Source: CAD feature listing. Evaluate the final solid. Frame: model axes, mm. Coordinates: 2 decimals unless noted, no trailing zeros. Order: outer loops, then holes, each group sorted by start corner. A loop starts at its lowest first (then second) coordinate and runs counter-clockwise, first axis right, second up.
Item 1: Contact query for flat-ended pins moving along their axis: P1, Ø12, axis at x = 364, y = -477, coming from the +Z side; P2, Ø1, axis at x = 401.5, z = 6, coming from the -Y side; P3, Ø12, axis at x = 375.5, z = 83.5, coming from the +Y side. Output: stop coordinate, or through.
Item 2: Ray query, line 1 (Z direction, x = 364.5, y = 584); line 2 (Y direction, x = 385, z = 88); line 3 (Y direction, x = 375, z = 37). Return the intervals inside material, ascending.
Item 3: Mould query, pull axis Y, two halves, no side actions, for faces 1 (the flat face through (376, 816, 0)), 2 (the cylindrical face through (360.89, 829.51, 50.09)), 3 (the cylindrical face through (387.09, 794.28, 50.09)), 4 (the flat face through (356, 821, 101.6)). Classes: released by +Y, released by -Y, zero draft, split by the parting line, or undercut.
Item 4: Section A-A on x = 370. Return the cut outline in (y, z).
Item 5: Section B-B on y = 584.5. Return the cut outline in (x, z), then the cut area to 3 significant figures.
Item 6: Section C-C on z = 19. Return the cut outline in (x, y), then the cut area to 3 significant figures.
from build123d import *

# Parameters (mm, degrees)
F0_W     = 76.2
F0_H     = 2133.6
F1_DEPTH = 4.7625
F2_R     = 24.13
F2_R_2   = 20.447
F3_DEPTH = 101.6
F5_DEPTH = 35.814


with BuildPart() as f1:
    # F0 (on Top) → F1 (new body)
    with BuildSketch(Plane.XY):
        with Locations((375.958569, -213.009804)):
            Rectangle(F0_W, F0_H)
    extrude(amount=-F1_DEPTH)

    # F2 (on face) → F3 (join)
    with BuildSketch(Plane.XY):
        with Locations((375.958569, 815.690196)):
            Circle(F2_R)
        with Locations((375.958569, 815.690196)):
            Circle(F2_R_2, mode=Mode.SUBTRACT)
    extrude(amount=F3_DEPTH)

    # F4 (on face) → F5 (cut)
    with BuildSketch(Plane(origin=(0, 0, -4.7625), x_dir=(1, 0, 0), z_dir=(0, 0, -1))):
        Polygon((337.858569, 1107.854731), (414.058569, 1279.809804), (337.858569, 1279.809804), align=None)
    extrude(amount=-F5_DEPTH, mode=Mode.SUBTRACT)


solid = f1.part
Answer list:
1. P1: stops at z = 0
1. P2: passes through
1. P3: stops at y = 839.82
2. line 1: z = -4.76 to 0
2. line 2: y = 793.32 to 797.35, 834.03 to 838.06
2. line 3: y = 791.58 to 795.27, 836.11 to 839.8
3. face 1: undercut
3. face 2: undercut
3. face 3: split by the parting line
3. face 4: zero draft
4. outline: (-1180.39, -4.76) - (853.79, -4.76) - (853.79, 0) - (839.07, 0) - (839.07, 101.6) - (835.25, 101.6) - (835.25, 0) - (796.13, 0) - (796.13, 101.6) - (792.31, 101.6) - (792.31, 0) - (-1180.39, 0) - close
5. outline: (337.86, -4.76) - (414.06, -4.76) - (414.06, 0) - (337.86, 0) - close
5. area: 363 mm2
6. outline: circle Ø48.26 at (375.96, 815.69); hole circle Ø40.89 at (375.96, 815.69)
6. area: 516 mm2
